Here's how the part is built. I have some questions about the finished solid (model axes, mm). Face numbers are marked on the shaded views. A direction names the side the tool comes from. Round coordinates to 2 decimals unless told otherwise and drop trailing zeros. Order: outer loops, then holes, each group sorted by start corner. A loop starts at its lowest first (then second) coordinate and runs counter-clockwise, first axis right, second up. Notation, with made-up numbers: M 7,50.5 L 28,50.5 A20 ccw 28,76.5 Z; hole C 9,-39.5 d3. An arc over 180 degrees is marked long. Write item = value, one per line. Start each with the question number.
Item 1: I want a section at C-C, the plane z = 45.5. List the corners of the cut face in (x, y) for me (3 decimals), plus the area to 3 significant figures.
Item 2: Please list where these lines run through material, in increasing order: L1, parallel to X at y = -17.25, z = -31.5 (3 decimals); L2, parallel to X at y = 3.75, z = 32 (3 decimals); L3, parallel to X at y = -1.75, z = 37.
Item 3: For the marked faces 4 and 5, which set-ups out of +Z, -Z, +X, -X, +Y, -Y let a thin tool reach every point of the face, with its end or its side?
Item 4: I'm going to push flat-ended pins straight in: P1, Ø22.5, axis at x = -69.5, z = 47, coming from the +Y side; P2, Ø4, axis at x = -39.5, y = 2.5, coming from the +Z side; P3, Ø12.5, axis at x = 50.5, y = -10, coming from the -Z side. Where does each tip first touch, or does it pass through?
Item 5: We'd pull the mould along Z, two halves only. Please class the marked faces 1, 2 and 3: pulls with the +Z half, pulls with the -Z half, needs draft (parallel to the pull), parting line crosses it, or undercut.
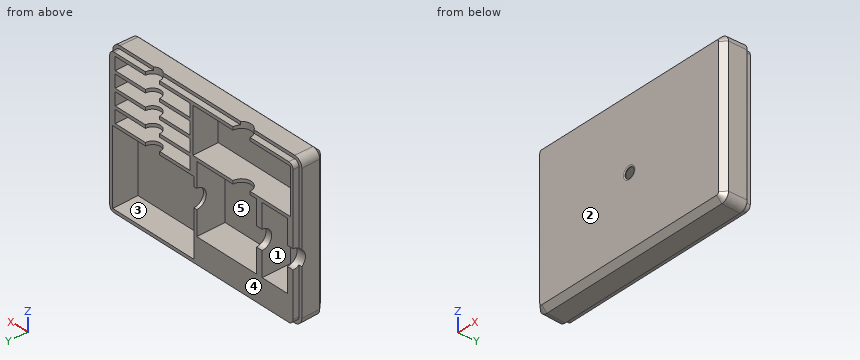
```python
from build123d import *
from OCP.BRepFilletAPI import BRepFilletAPI_MakeChamfer

# Parameters (mm, degrees)
BOSS_EXTRUDE1_DEPTH            = 23.495
BOSS_EXTRUDE1_DRAFT            = -1.5
CHAMFER1_SIZE                  = 5.21838973
CHAMFER1_SIZE_2                = 5.08
BOSS_EXTRUDE2_DEPTH            = 5.842
SKETCH3_W                      = 108.712
SKETCH3_H                      = 45.212
CUT_EXTRUDE1_DEPTH             = 25.4
SKETCH4_R                      = 6.35
CUT_EXTRUDE2_DEPTH             = 1.524
CHAMFER2_SIZE2                 = 4.064
CHAMFER2_SIZE                  = 1.524
SKETCH5_W                      = 28.194
SKETCH5_H                      = 67.564
SKETCH5_W_2                    = 66.548
CUT_EXTRUDE3_DEPTH             = 28.194
SKETCH6_W                      = 83.312
SKETCH6_H                      = 12.7
CUT_EXTRUDE4_DEPTH             = 25.4
LPATTERN2_COUNT                = 4
LPATTERN2_PITCH                = 15.875
SKETCH8_W                      = 90.678
SKETCH8_H                      = 74.422
CUT_EXTRUDE5_DEPTH             = 25.4
CUT_EXTRUDE6_REACH             = 148.547
SKETCH10_R                     = 9.525
CUT_EXTRUDE6_DIRECTION_2_REACH = 148.547
SKETCH11_R                     = 9.525
CUT_EXTRUDE7_DEPTH             = 185.471292474
CUT_EXTRUDE7_DIRECTION_2_REACH = 186.471
CUT_EXTRUDE8_REACH             = 172.219
CUT_EXTRUDE8_DIRECTION_2_DEPTH = 171.218901151
SKETCH12_R                     = 5.067701835
CUT_EXTRUDE9_DEPTH             = 133.581735005


with BuildPart() as part:
    # Sketch1 → Boss-Extrude1 (with draft: the straight prism first)
    with BuildSketch(Plane(origin=(0, 0, 0), x_dir=(1, 0, 0), z_dir=(0, 1, 0))):
        with BuildLine():
            ThreePointArc((-97.4725, 75.311), (-103.085160076, 72.986160076), (-105.41, 67.3735))
            Line((-105.41, 67.3735), (-105.41, -67.3735))
            ThreePointArc((-105.41, -67.3735), (-103.085160076, -72.986160076), (-97.4725, -75.311))
            Line((-97.4725, -75.311), (97.4725, -75.311))
            ThreePointArc((97.4725, -75.311), (103.085160076, -72.986160076), (105.41, -67.3735))
            Line((105.41, -67.3735), (105.41, 67.3735))
            ThreePointArc((105.41, 67.3735), (103.085160076, 72.986160076), (97.4725, 75.311))
            Line((97.4725, 75.311), (-97.4725, 75.311))
        make_face()
    extrude(amount=-BOSS_EXTRUDE1_DEPTH)
    # Boss-Extrude1: the draft: its side faces are tilted about the plane it starts from
    boss_extrude1_sides = [part.faces().sort_by_distance(p)[0] for p in [
        (-103.085160076, -11.7475, -72.986160076),
        (-105.41, -11.7475, 0),
        (-103.085160076, -11.7475, 72.986160076),
        (0, -11.7475, 75.311),
        (103.085160076, -11.7475, 72.986160076),
        (105.41, -11.7475, 0),
        (103.085160076, -11.7475, -72.986160076),
        (0, -11.7475, -75.311),
    ]]
    draft(boss_extrude1_sides, Plane(origin=(0, 0, 0), x_dir=(1, 0, 0), z_dir=(0, 1, 0)), BOSS_EXTRUDE1_DRAFT)

    # Chamfer1
    chamfer1_edges_1 = [part.edges().sort_by_distance(p)[0] for p in [
        (-102.650120953, -23.495, -72.551120953),
    ]]
    chamfer1_side_1 = [part.faces().sort_by_distance(p)[0] for p in [
        (-102.652001559, -23.393434816, -72.553001559),
    ]]
    chamfer1_edges_2 = [part.edges().sort_by_distance(p)[0] for p in [
        (-104.794761773, -23.495, 0),
    ]]
    chamfer1_side_2 = [part.faces().sort_by_distance(p)[0] for p in [
        (-104.797421351, -23.393434816, 0),
    ]]
    chamfer1_edges_3 = [part.edges().sort_by_distance(p)[0] for p in [
        (-102.650120953, -23.495, 72.551120953),
    ]]
    chamfer1_side_3 = [part.faces().sort_by_distance(p)[0] for p in [
        (-102.652001559, -23.393434816, 72.553001559),
    ]]
    chamfer1_edges_4 = [part.edges().sort_by_distance(p)[0] for p in [
        (0, -23.495, 74.695761773),
    ]]
    chamfer1_side_4 = [part.faces().sort_by_distance(p)[0] for p in [
        (0, -23.393434816, 74.698421351),
    ]]
    chamfer1_edges_5 = [part.edges().sort_by_distance(p)[0] for p in [
        (102.650120953, -23.495, 72.551120953),
    ]]
    chamfer1_side_5 = [part.faces().sort_by_distance(p)[0] for p in [
        (102.652001559, -23.393434816, 72.553001559),
    ]]
    chamfer1_edges_6 = [part.edges().sort_by_distance(p)[0] for p in [
        (104.794761773, -23.495, 0),
    ]]
    chamfer1_side_6 = [part.faces().sort_by_distance(p)[0] for p in [
        (104.797421351, -23.393434816, 0),
    ]]
    chamfer1_edges_7 = [part.edges().sort_by_distance(p)[0] for p in [
        (102.650120953, -23.495, -72.551120953),
    ]]
    chamfer1_side_7 = [part.faces().sort_by_distance(p)[0] for p in [
        (102.652001559, -23.393434816, -72.553001559),
    ]]
    chamfer1_edges_8 = [part.edges().sort_by_distance(p)[0] for p in [
        (0, -23.495, -74.695761773),
    ]]
    chamfer1_side_8 = [part.faces().sort_by_distance(p)[0] for p in [
        (0, -23.393434816, -74.698421351),
    ]]
    chamfer1 = BRepFilletAPI_MakeChamfer(part.part.solid().wrapped)
    for e in chamfer1_edges_1:
        chamfer1.Add(CHAMFER1_SIZE, CHAMFER1_SIZE_2, e.wrapped, chamfer1_side_1[0].wrapped)
    for e in chamfer1_edges_2:
        chamfer1.Add(CHAMFER1_SIZE, CHAMFER1_SIZE_2, e.wrapped, chamfer1_side_2[0].wrapped)
    for e in chamfer1_edges_3:
        chamfer1.Add(CHAMFER1_SIZE, CHAMFER1_SIZE_2, e.wrapped, chamfer1_side_3[0].wrapped)
    for e in chamfer1_edges_4:
        chamfer1.Add(CHAMFER1_SIZE, CHAMFER1_SIZE_2, e.wrapped, chamfer1_side_4[0].wrapped)
    for e in chamfer1_edges_5:
        chamfer1.Add(CHAMFER1_SIZE_2, CHAMFER1_SIZE, e.wrapped, chamfer1_side_5[0].wrapped)
    for e in chamfer1_edges_6:
        chamfer1.Add(CHAMFER1_SIZE, CHAMFER1_SIZE_2, e.wrapped, chamfer1_side_6[0].wrapped)
    for e in chamfer1_edges_7:
        chamfer1.Add(CHAMFER1_SIZE, CHAMFER1_SIZE_2, e.wrapped, chamfer1_side_7[0].wrapped)
    for e in chamfer1_edges_8:
        chamfer1.Add(CHAMFER1_SIZE, CHAMFER1_SIZE_2, e.wrapped, chamfer1_side_8[0].wrapped)
    add(Compound.cast(chamfer1.Shape()), mode=Mode.REPLACE)

    # Sketch2 → Boss-Extrude2 (add)
    with BuildSketch(Plane(origin=(0, 0, 0), x_dir=(1, 0, 0), z_dir=(0, 1, 0))):
        with BuildLine():
            Line((97.4725, 72.136), (-97.4725, 72.136))
            ThreePointArc((-97.4725, 72.136), (-100.840096045, 70.741096045), (-102.235, 67.3735))
            Line((-102.235, 67.3735), (-102.235, -67.3735))
            ThreePointArc((-102.235, -67.3735), (-100.840096045, -70.741096045), (-97.4725, -72.136))
            Line((-97.4725, -72.136), (97.4725, -72.136))
            ThreePointArc((97.4725, -72.136), (100.840096045, -70.741096045), (102.235, -67.3735))
            Line((102.235, -67.3735), (102.235, 67.3735))
            ThreePointArc((102.235, 67.3735), (100.840096045, 70.741096045), (97.4725, 72.136))
        make_face()
    extrude(amount=BOSS_EXTRUDE2_DEPTH)

    # Sketch3 → Cut-Extrude1 (cut)
    with BuildSketch(Plane(origin=(0, 5.842, 0), x_dir=(1, 0, 0), z_dir=(0, 1, 0))):
        with Locations((-44.704, -46.355)):
            Rectangle(SKETCH3_W, SKETCH3_H)
    extrude(amount=-CUT_EXTRUDE1_DEPTH, mode=Mode.SUBTRACT)

    # Sketch4 → Cut-Extrude2 (cut)
    with BuildSketch(Plane.XZ.offset(23.495)):
        with Locations(Location((0, 0, 0), (0, 0, 270))):
            Circle(SKETCH4_R)
    extrude(amount=-CUT_EXTRUDE2_DEPTH, mode=Mode.SUBTRACT)

    # Chamfer2
    chamfer2_edges = [part.edges().sort_by_distance(p)[0] for p in [
        (0, -21.971, 6.35),
    ]]
    chamfer2_side = [part.faces().sort_by_distance(p)[0] for p in [
        (0, -22.00148, 6.35),
    ]]
    chamfer(chamfer2_edges, length=CHAMFER2_SIZE - 0.0001, length2=CHAMFER2_SIZE2 - 0.0001, reference=chamfer2_side[0])  # a hair under: the kernel refuses the full size

    # Sketch5 → Cut-Extrude3 (cut)
    with BuildSketch(Plane(origin=(0, 5.842, 0), x_dir=(1, 0, 0), z_dir=(0, 1, 0))):
        with Locations((-81.788, 13.208)):
            Rectangle(SKETCH5_W, SKETCH5_H)
        with Locations((-28.067, 13.208)):
            Rectangle(SKETCH5_W_2, SKETCH5_H)
    extrude(amount=-CUT_EXTRUDE3_DEPTH, mode=Mode.SUBTRACT)

    # Sketch6 → Cut-Extrude4 (cut)
    with BuildSketch(Plane(origin=(0, 5.842, 0), x_dir=(1, 0, 0), z_dir=(0, 1, 0))):
        with Locations((54.483, -62.611)):
            Rectangle(SKETCH6_W, SKETCH6_H)
    cut_extrude4 = extrude(amount=-CUT_EXTRUDE4_DEPTH, mode=Mode.SUBTRACT)

    # LPattern2: Cut-Extrude4 ×4
    with Locations(*[(0, 0, -i * LPATTERN2_PITCH) for i in range(1, LPATTERN2_COUNT)]):
        add(cut_extrude4, mode=Mode.SUBTRACT)

    # Sketch8 → Cut-Extrude5 (cut)
    with BuildSketch(Plane(origin=(0, 5.842, 0), x_dir=(1, 0, 0), z_dir=(0, 1, 0))):
        with Locations((53.721, 31.75)):
            Rectangle(SKETCH8_W, SKETCH8_H)
    extrude(amount=-CUT_EXTRUDE5_DEPTH, mode=Mode.SUBTRACT)

    # Sketch10 → Cut-Extrude6 (cut, up to next)
    with BuildSketch(Plane.XY.offset(23.749), mode=Mode.PRIVATE) as cut_extrude6_sk1:
        with Locations((-44.704, 5.842)):
            Circle(SKETCH10_R)
    cut_extrude6_tool1 = extrude(cut_extrude6_sk1.sketch, amount=-CUT_EXTRUDE6_REACH, mode=Mode.PRIVATE) & part.part
    add(cut_extrude6_tool1.solids().sort_by_distance((-44.704, 5.842, 23.749))[0], mode=Mode.SUBTRACT)

    # Sketch10 → Cut-Extrude6 direction 2 (cut, up to next)
    with BuildSketch(Plane.XY.offset(23.749), mode=Mode.PRIVATE) as cut_extrude6_direction_2_sk1:
        with Locations((-44.704, 5.842)):
            Circle(SKETCH10_R)
    cut_extrude6_direction_2_tool1 = extrude(cut_extrude6_direction_2_sk1.sketch, amount=CUT_EXTRUDE6_DIRECTION_2_REACH, mode=Mode.PRIVATE) & part.part
    add(cut_extrude6_direction_2_tool1.solids().sort_by_distance((-44.704, 5.842, 23.749))[0], mode=Mode.SUBTRACT)

    # Sketch11 → Cut-Extrude7 (cut)
    with BuildSketch(Plane(origin=(-61.341, 0, 0), x_dir=(0, 0, -1), z_dir=(1, 0, 0))):
        with Locations((13.208, 5.842)):
            Circle(SKETCH11_R)
    extrude(amount=-CUT_EXTRUDE7_DEPTH, mode=Mode.SUBTRACT)

    # Sketch11 → Cut-Extrude7 direction 2 (cut, up to next)
    with BuildSketch(Plane(origin=(-61.341, 0, 0), x_dir=(0, 0, -1), z_dir=(1, 0, 0)), mode=Mode.PRIVATE) as cut_extrude7_direction_2_sk1:
        with Locations((13.208, 5.842)):
            Circle(SKETCH11_R)
    cut_extrude7_direction_2_tool1 = extrude(cut_extrude7_direction_2_sk1.sketch, amount=CUT_EXTRUDE7_DIRECTION_2_REACH, mode=Mode.PRIVATE) & part.part
    add(cut_extrude7_direction_2_tool1.solids().sort_by_distance((-61.341, 5.842, -13.208))[0], mode=Mode.SUBTRACT)

    # Cut-Extrude8: up to this face of the body (flat: up to its plane)
    cut_extrude8_end = Plane(part.part.faces().sort_by_distance((53.721, -6.858, 5.461))[0])
    # Sketch7 → Cut-Extrude8 (cut, up to the picked face)
    with BuildSketch(Plane.XY.offset(56.261), mode=Mode.PRIVATE) as cut_extrude8_sk1:
        with BuildLine():
            Line((46.5455, 5.842), (54.483, 5.842))
            Line((54.483, 5.842), (62.4205, 5.842))
            ThreePointArc((62.4205, 5.842), (54.483, -2.0955), (46.5455, 5.842))
        make_face()
    cut_extrude8_tool1 = split(extrude(cut_extrude8_sk1.sketch, amount=-CUT_EXTRUDE8_REACH, mode=Mode.PRIVATE), bisect_by=cut_extrude8_end, keep=Keep.BOTH, mode=Mode.PRIVATE)
    add(cut_extrude8_tool1.solids().sort_by(Axis((54.483, 2.47322, 56.261), (0, 0, -1)))[0], mode=Mode.SUBTRACT)

    # Sketch7 → Cut-Extrude8 direction 2 (cut)
    with BuildSketch(Plane.XY.offset(56.261)):
        with BuildLine():
            Line((46.5455, 5.842), (54.483, 5.842))
            Line((54.483, 5.842), (62.4205, 5.842))
            ThreePointArc((62.4205, 5.842), (54.483, -2.0955), (46.5455, 5.842))
        make_face()
    extrude(amount=CUT_EXTRUDE8_DIRECTION_2_DEPTH, mode=Mode.SUBTRACT)

    # Sketch12 → Cut-Extrude9 (cut, through all)
    with BuildSketch(Plane(origin=(0, -22.352, 0), x_dir=(1, 0, 0), z_dir=(0, 1, 0))):
        with Locations(Location((0, 0, 0), (0, 0, 270))):
            Circle(SKETCH12_R)
    extrude(amount=-CUT_EXTRUDE9_DEPTH, mode=Mode.SUBTRACT)


solid = part.part
```
Filled in:
q1.outline = M -105.41,0 L -104.931,-18.278 L -99.715,-23.495 L 99.715,-23.495 L 104.931,-18.278 L 105.41,0 L 102.235,0 L 102.235,5.842 L 96.139,5.842 L 96.139,-19.558 L 12.827,-19.558 L 12.827,5.842 L 9.652,5.842 L 9.652,-19.558 L -99.06,-19.558 L -99.06,5.842 L -102.235,5.842 L -102.235,0 Z
q1.area = 1,230 mm^2
q2.L1 = -104.958 to -95.885, -67.691 to -61.341, 5.207 to 8.382, 99.06 to 104.958
q2.L2 = -102.235 to -99.06, 9.652 to 12.827, 96.139 to 102.235
q2.L3 = -105.36 to -99.06, 9.65 to 12.83, 96.14 to 105.36
q3.face_4 = +Z, -Z, +X, -X, +Y
q3.face_5 = +Y
q4.P1 = -19.56
q4.P2 = -46.99
q4.P3 = -75.21
q5.face_1 = undercut
q5.face_2 = needs draft
q5.face_3 = undercut
